Read the model definition and answer for the solid it produces. Units are mm, in the model's axes. Coordinates: 2 decimals unless noted, no trailing zeros. Loops run counter-clockwise (first coordinate to the right, second up) from the corner with the lowest first, then second, coordinate; pieces in that order, holes last.
Q1. The mould has two halves that part along X. Classify faces 1 (the face through (73.72, 42.31, 1.97)), 2 (the face through (-0.99, 5.74, 1.97)), 3 (the face through (31, 18, 4)): pulls with the +X half, pulls with the -X half, needs draft (parallel to the pull), parting line crosses it, or undercut.
Q2. Straight lines are drawn through the part: line 1 (Y direction, x = 0, z = 1.65); line 2 (Y direction, x = 63, z = 3.65); line 3 (Y direction, x = 2.5, z = 2.35). For each, find the intervals that lie inside material, in ascending order.
Q3. Section A-A (x = 0) is taken. Give the vertices of the cut face in (y, z).
Q4. Section B-B (z = 1.55) is taken. Give the vertices of the cut face in (x, y).
Q5. Section D-D (x = 65) is taken. Give the vertices of the cut face in (y, z), then the cut area to 3 significant figures.
Q6. Flat-ended cylindrical pins translate along their axes: P1, Ø2, axis at x = -5.63, y = -3.25, coming from the +Z side; P2, Ø3, axis at x = 0, y = 6.51, coming from the -Z side; P3, Ø1, axis at x = 35.5, z = 2.5, coming from the -Y side; P4, Ø1, axis at x = 50, z = 1.5, coming from the +Y side. Find the tip coordinate at first contact, or state that the pin passes through.
Q7. Section C-C (y = 0) is taken. Give the vertices of the cut face in (x, z), then the cut area to 3 significant figures.
from build123d import *

# Parameters (mm, degrees)
SKETCH1_R           = 12.5
SKETCH1_R_2         = 4
SKETCH1_R_3         = 1.25
SKETCH1_R_4         = 10
SKETCH1_R_5         = 2.5
BOSS_EXTRUDE1_DEPTH = 4


with BuildPart() as part:
    # Sketch1 → Boss-Extrude1 (new body)
    # profile 1 of 3: a face of its own
    with BuildSketch(Plane.XY):
        Circle(SKETCH1_R)
        Circle(SKETCH1_R_2, mode=Mode.SUBTRACT)
        with Locations((0, 6.505402357)):
            Circle(SKETCH1_R_3, mode=Mode.SUBTRACT)
        with Locations((5.633843703, -3.252701179)):
            Circle(SKETCH1_R_3, mode=Mode.SUBTRACT)
        with Locations((-5.633843703, -3.252701179)):
            Circle(SKETCH1_R_3, mode=Mode.SUBTRACT)
    # profile 2 of 3: a face of its own
    with BuildSketch(Plane.XY):
        with BuildLine():
            ThreePointArc((70.237801869, 29.011225218), (56.291651246, 32.5), (60.243358968, 46.322108115))
            Line((60.243358968, 46.322108115), (-5.885682894, 11.027635144))
            ThreePointArc((-5.885682894, 11.027635144), (6.429578673, 10.719632367), (12.5, 0))
            ThreePointArc((12.5, 0), (10.92799465, -6.068684613), (6.607370731, -10.610968477))
            Line((6.607370731, -10.610968477), (70.237801869, 29.011225218))
        make_face()
    # profile 3 of 3: a face of its own
    with BuildSketch(Plane.XY):
        with Locations((64.951905284, 37.5)):
            Circle(SKETCH1_R_4)
        with Locations((64.951905284, 37.5)):
            Circle(SKETCH1_R_5, mode=Mode.SUBTRACT)
    extrude(amount=BOSS_EXTRUDE1_DEPTH)


solid = part.part
Numbers:
1. face 1: parting line crosses it
1. face 2: undercut
1. face 3: needs draft
2. line 1: y = -12.5 to -4, 4 to 5.26, 7.76 to 14.17
2. line 2: y = 24.5 to 35.94, 39.06 to 47.31
2. line 3: y = -12.25 to -3.12, 3.12 to 15.5
3. outline: (-12.5, 0) - (-4, 0) - (-4, 4) - (-12.5, 4) - close; (4, 0) - (5.26, 0) - (5.26, 4) - (4, 4) - close; (7.76, 0) - (14.17, 0) - (14.17, 4) - (7.76, 4) - close
4. outline: (-5.89, 11.03) arc R12.5 ccw (long way) to (6.61, -10.61) - (70.24, 29.01) arc R10 ccw to (60.24, 46.32) - close; hole circle Ø2.5 at (-5.63, -3.25); hole circle Ø8 at (0, 0); hole circle Ø2.5 at (0, 6.51); hole circle Ø2.5 at (5.63, -3.25); hole circle Ø5 at (64.95, 37.5)
5. outline: (25.75, 0) - (35, 0) - (35, 4) - (25.75, 4) - close; (40, 0) - (47.5, 0) - (47.5, 4) - (40, 4) - close
5. area: 67.0 mm2
6. P1: passes through
6. P2: stops at z = 0
6. P3: stops at y = 7.07
6. P4: stops at y = 41.12
7. outline: (-12.5, 0) - (-4, 0) - (-4, 4) - (-12.5, 4) - close; (4, 0) - (23.65, 0) - (23.65, 4) - (4, 4) - close
7. area: 113 mm2
